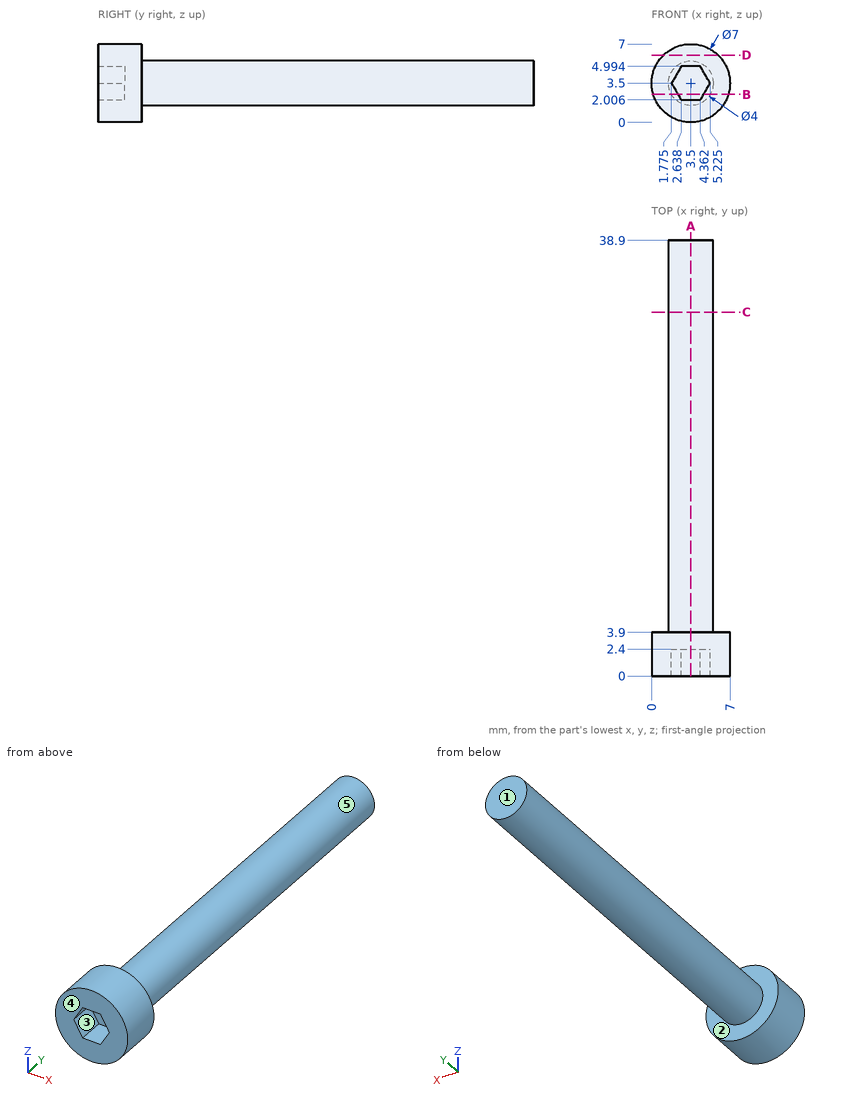
Can you work these out from the drawing? Everything is in mm from the part's minimum corner. A direction names the side the tool comes from. Coordinates: 2 decimals unless noted, no trailing zeros. Loops run counter-clockwise (first coordinate to the right, second up) from the corner with the lowest first, then second, coordinate; pieces in that order, holes last. Notation, with made-up numbers: M 42.5,24 L 70.5,24 A7 cw 70.5,37 Z; hole C 74.5,6.5 d1. An arc over 180 degrees is marked long. Put each result on its own line as item: value. Start each with the question number.
(1) Will these pins go through, and if not, where does the flat tip stop? P1, Ø0.9, axis at x = 4, y = 1, coming from the +Z side; P2, Ø1.5, axis at x = 5, y = 26.5, coming from the -Z side (1 decimal); P3, Ø1.5, axis at x = 4, z = 3.5, coming from the -Y side; P4, Ø1.5, axis at x = 4, y = 18.5, coming from the +Z side.
(2) I need wall thicknesses on line 1 (Y direction, x = 5.5, z = 2.25); line 2 (Z direction, x = 2.5, y = 6). Which ranges of each line are inside material? Lowest first, please. Write a range as from..to.
(3) Suppose I cut it at C-C on y = 32.5. Please give me the cut outline in (x, z).
(4) Thinking about a two-plate mould opening in X: for the marked faces 3, 4 and 5, which applies, pulls with the +X half, pulls with the -X half, needs draft (parallel to the pull), parting line crosses it, or undercut?
(5) Suppose I cut it at D-D on z = 6. Please give me the cut outline in (x, y).
(6) Suppose I cut it at A-A on x = 3.5. Please give me the cut outline in (y, z).
(7) Suppose I cut it at B-B on z = 2.5. Please give me the cut outline in (x, y) (1 decimal).
(8) For the marked faces 1 and 2, which set-ups out of +Z, -Z, +X, -X, +Y, -Y let a thin tool reach every point of the face, with its end or its side?
Solutions:
1. P1: stops at z = 7
1. P2: stops at z = 1.6
1. P3: stops at y = 2.4
1. P4: stops at z = 5.5
2. line 1: y = 0..3.9
2. line 2: z = 1.77..5.23
3. outline: C 3.5,3.5 d4
4. face 3: undercut
4. face 4: needs draft
4. face 5: parting line crosses it
5. outline: M 1.05,0 L 5.95,0 L 5.95,3.9 L 1.05,3.9 Z
6. outline: M 0,0 L 3.9,0 L 3.9,1.5 L 38.9,1.5 L 38.9,5.5 L 3.9,5.5 L 3.9,7 L 0,7 L 0,4.99 L 2.4,4.99 L 2.4,2.01 L 0,2.01 Z
7. outline: M 0.1,0 L 2.4,0 L 2.4,2.4 L 4.6,2.4 L 4.6,0 L 6.9,0 L 6.9,3.9 L 5.2,3.9 L 5.2,38.9 L 1.8,38.9 L 1.8,3.9 L 0.1,3.9 Z
8. face 1: +Z, -Z, +X, -X, +Y
8. face 2: +Y
